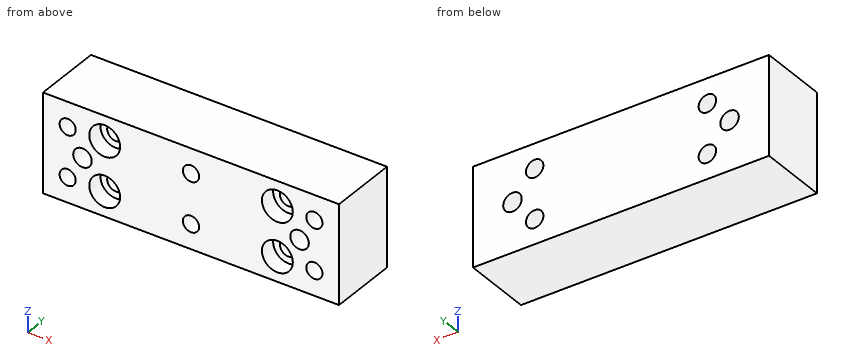
```python
from build123d import *

# Parameters (mm, degrees)
F0_W           = 76.2
F0_H           = 25.4
F1_DEPTH       = 17.78
F3_D           = 4.1656
F3_DEPTH       = 8.382
F3_TIP         = 1.2514724973
F5_D           = 4.4958
F5_CBORE_D     = 7.9502
F5_CBORE_DEPTH = 4.1656
F7_D           = 4.7625


with BuildPart() as f1:
    # F0 (on Front) → F1 (new body)
    with BuildSketch(Plane.XZ):
        Rectangle(F0_W, F0_H)
    extrude(amount=F1_DEPTH)

    # F3
    with Locations(Plane.XZ.offset(17.78)):
        with Locations((-31.75, 6.35), (0, 6.35), (31.75, 6.35), (31.75, -6.35), (0, -6.35), (-31.75, -6.35)):
            Hole(F3_D / 2, depth=F3_DEPTH)
            with Locations((0, 0, -(F3_DEPTH + F3_TIP / 2))):  # 118° drill point
                Cone(0, F3_D / 2, F3_TIP, mode=Mode.SUBTRACT)

    # F5 (through all)
    with Locations(Plane.XZ.offset(17.78)):
        with Locations((-22.225, 6.35), (22.225, 6.35), (22.225, -6.35), (-22.225, -6.35)):
            CounterBoreHole(F5_D / 2, F5_CBORE_D / 2, F5_CBORE_DEPTH)

    # F7 (through all)
    with Locations(Plane.XZ.offset(17.78)):
        with Locations((-27.94, 0), (27.94, 0)):
            Hole(F7_D / 2)


solid = f1.part
```
Check sheet for the modelled part. Datum: model origin and axes. Units: mm. Give positions to 0.01 mm unless a question says otherwise; leave off trailing zeros. Write each loop counter-clockwise with the first axis right and the second up, starting at its lowest first coordinate (ties: lowest second). Pieces come first, ordered by that corner, then holes. Notation, with made-up numbers: (44, 56.25) - (91, 56.25) arc R15 cw to (91, 85.25) - close; hole circle Ø9 at (84, -7.5). An arc over 180 degrees is marked (long way). Answer as a JSON object with one key per item and string values. Group by question number.
1) Thickness scan on probe 1 along Z at (x, y) = (-31.75, -13); probe 2 along X at (y, z) = (-9.75, -6.25); probe 3 along X at (y, z) = (-17, 4.75). Record the ranges inside material, lowest first. Write a range as from..to.
2) Depth check by flat-ended pin: P1, Ø2.5, axis at x = -22.225, z = -6.35, coming from the +Y side; P2, Ø6.5, axis at x = 22.225, z = 6.35, coming from the -Y side; P3, Ø2.5, axis at x = 31.75, z = -6.35, coming from the -Y side; P4, Ø3.5, axis at x = -31.75, z = 6.35, coming from the -Y side. Enter the tip coordinate at first touch or a pass-through.
3) Sectioned sample at A-A (x = -27.94). Record the cut outline in (y, z).
4) Sectioned sample at B-B (y = -2.75). Give the number of separate pieces and of enclosed holes in the cut face, then the cut area to 3 significant figures.
5) Sectioned sample at C-C (z = 0). Record the cut outline in (x, y).
Geometry results:
{
 "1": {"probe 1": "z = -12.7..-8.43, -4.27..4.27, 8.43..12.7", "probe 2": "x = -38.1..-33.83, -29.67..-24.47, -19.98..-2.08, 2.08..19.98, 24.47..29.67, 33.83..38.1", "probe 3": "x = -38.1..-33.08, -30.42..-25.86, -18.59..-1.33, 1.33..18.59, 25.86..30.42, 33.08..38.1"},
 "2": {"P1": "passes through", "P2": "stops at y = -13.61", "P3": "stops at y = -8.9", "P4": "stops at y = -9.2"},
 "3": {"outline": "(-17.78, -12.7) - (0, -12.7) - (0, -2.38) - (-17.78, -2.38) - close; (-17.78, 2.38) - (0, 2.38) - (0, 12.7) - (-17.78, 12.7) - close"},
 "4": {"separate pieces": "1", "enclosed holes": "6", "area": "1,840 mm^2"},
 "5": {"outline": "(-38.1, -17.78) - (-30.32, -17.78) - (-30.32, 0) - (-38.1, 0) - close; (-25.56, -17.78) - (25.56, -17.78) - (25.56, 0) - (-25.56, 0) - close; (30.32, -17.78) - (38.1, -17.78) - (38.1, 0) - (30.32, 0) - close"}
}
